Geometry check sheet. Reference: the model listing, model coordinates, mm. Coordinates: 2 decimals unless noted, no trailing zeros. Order: outer loops, then holes, each group sorted by start corner. A loop starts at its lowest first (then second) coordinate and runs counter-clockwise, first axis right, second up. Notation, with made-up numbers: (85.5, 7.5) - (129.5, 7.5) arc R31 cw to (129.5, 40.5) - close; hole circle Ø8 at (-37.75, 20). An arc over 180 degrees is marked (long way). Use CSV: the item, a comma, the result in double quotes. Start each with the question number.
1) Sectioned sample at A-A, the plane z = 7. Count the separate pieces of the cut face and the enclosed holes in it, and give its area (3 significant figures).
2) Depth check by flat-ended pin: P1, Ø1.9, axis at y = 668, z = 7.5, coming from the -X side; P2, Ø3.5, axis at x = -10.32, y = 357.19, coming from the -Z side; P3, Ø3, axis at x = 34.5, z = 3, coming from the +Y side; P4, Ø2, axis at x = -44, z = 10.5, coming from the +Y side. Enter the tip coordinate at first touch or a pass-through.
3) Sectioned sample at B-B, the plane y = 82.5. Record the cut outline in (x, z) (3 decimals), and give its area (3 significant figures).
4) Thickness scan on probe 1 along Y at (x, z) = (-18, 10); probe 2 along X at (y, z) = (237, 3) (3 decimals); probe 3 along X at (y, z) = (62, 6.25). Record the ranges inside material, lowest first. Write a range as [from, to].
from build123d import *

# Parameters (mm, degrees)
F1_DEPTH = 12.7
F2_SIZE  = 3.175
F3_R     = 2.15265
F4_DEPTH = 12.7


with BuildPart() as f1:
    # F0 (on Top) → F1 (new body)
    with BuildSketch(Plane.XY):
        with BuildLine():
            Line((-38.1, 38.1), (-38.1, 0))
            ThreePointArc((-38.1, 0), (0, -38.1), (38.1, 0))
            Line((38.1, 0), (38.1, 38.1))
            ThreePointArc((38.1, 38.1), (39.550095, 45.390119), (43.679616, 51.570384))
            Line((43.679616, 51.570384), (92.30064, 100.191409))
            ThreePointArc((92.30064, 100.191409), (99.183175, 110.49185), (101.6, 122.642049))
            Line((101.6, 122.642049), (101.6, 563.157951))
            ThreePointArc((101.6, 563.157951), (99.183175, 575.30815), (92.30064, 585.608591))
            Line((92.30064, 585.608591), (43.679616, 634.229616))
            ThreePointArc((43.679616, 634.229616), (39.550095, 640.409881), (38.1, 647.7))
            Line((38.1, 647.7), (38.1, 685.8))
            ThreePointArc((38.1, 685.8), (0, 723.9), (-38.1, 685.8))
            Line((-38.1, 685.8), (-38.1, 647.7))
            ThreePointArc((-38.1, 647.7), (-39.550095, 640.409881), (-43.679616, 634.229616))
            Line((-43.679616, 634.229616), (-92.30064, 585.608591))
            ThreePointArc((-92.30064, 585.608591), (-99.183175, 575.30815), (-101.6, 563.157951))
            Line((-101.6, 563.157951), (-101.6, 122.642049))
            ThreePointArc((-101.6, 122.642049), (-99.183175, 110.49185), (-92.30064, 100.191409))
            Line((-92.30064, 100.191409), (-43.679616, 51.570384))
            ThreePointArc((-43.679616, 51.570384), (-39.550095, 45.390119), (-38.1, 38.1))
        make_face()
    extrude(amount=F1_DEPTH)

    # F2
    f2_edges = [f1.edges().sort_by_distance(p)[0] for p in [
        (-39.550095, 45.390119, 0),
        (-38.1, 19.05, 0),
        (0, -38.1, 0),
        (38.1, 19.05, 0),
        (39.550095, 45.390119, 0),
        (67.990128, 75.880896, 0),
        (99.183175, 110.49185, 0),
        (101.6, 342.9, 0),
        (99.183175, 575.30815, 0),
        (67.990128, 609.919104, 0),
        (39.550095, 640.409881, 0),
        (38.1, 666.75, 0),
        (0, 723.9, 0),
        (-38.1, 666.75, 0),
        (-39.550095, 640.409881, 0),
        (-67.990128, 609.919104, 0),
        (-99.183175, 575.30815, 0),
        (-101.6, 342.9, 0),
        (-99.183175, 110.49185, 0),
        (-67.990128, 75.880896, 0),
        (-39.550095, 45.390119, 12.7),
        (-38.1, 19.05, 12.7),
        (0, -38.1, 12.7),
        (38.1, 19.05, 12.7),
        (39.550095, 45.390119, 12.7),
        (67.990128, 75.880896, 12.7),
        (99.183175, 110.49185, 12.7),
        (101.6, 342.9, 12.7),
        (99.183175, 575.30815, 12.7),
        (67.990128, 609.919104, 12.7),
        (39.550095, 640.409881, 12.7),
        (38.1, 666.75, 12.7),
        (0, 723.9, 12.7),
        (-38.1, 666.75, 12.7),
        (-39.550095, 640.409881, 12.7),
        (-67.990128, 609.919104, 12.7),
        (-99.183175, 575.30815, 12.7),
        (-101.6, 342.9, 12.7),
        (-99.183175, 110.49185, 12.7),
        (-67.990128, 75.880896, 12.7),
    ]]
    chamfer(f2_edges, length=F2_SIZE)

    # F3 (on face) → F4 (cut, through all)
    with BuildSketch(Plane(origin=(0, 0, 0), x_dir=(1, 0, 0), z_dir=(0, 0, -1))):
        with Locations((10.31875, -700.0875)):
            Circle(F3_R)
        with Locations((10.31875, -671.5125)):
            Circle(F3_R)
        with Locations((-10.31875, -671.5125)):
            Circle(F3_R)
        with Locations((-10.31875, -700.0875)):
            Circle(F3_R)
        with Locations((10.31875, -55.402948)):
            Circle(F3_R)
        with Locations((10.31875, -26.827948)):
            Circle(F3_R)
        with Locations((-10.31875, -55.402948)):
            Circle(F3_R)
        with Locations((-10.31875, -26.827948)):
            Circle(F3_R)
        with Locations((10.31875, -357.1875)):
            Circle(F3_R)
        with Locations((10.31875, -328.6125)):
            Circle(F3_R)
        with Locations((-10.31875, -328.6125)):
            Circle(F3_R)
        with Locations((-10.31875, -357.1875)):
            Circle(F3_R)
    extrude(amount=-F4_DEPTH, mode=Mode.SUBTRACT)


solid = f1.part
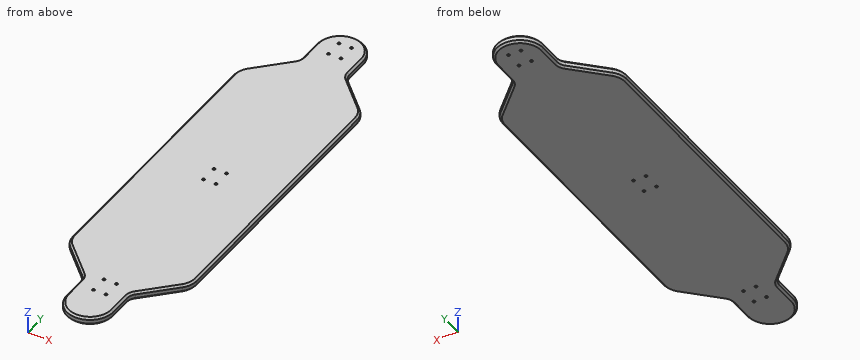
Evaluation:
1,separate pieces,"1"
1,enclosed holes,"12"
1,area,"124,000 mm²"
2,P1,"x = -38.1"
2,P2,"through"
2,P3,"y = 704.82"
2,P4,"y = 634.26"
3,outline,"(-74.609, 3.175) - (-70.119, 0) - (70.119, 0) - (74.609, 3.175) - (74.609, 9.525) - (70.119, 12.7) - (-70.119, 12.7) - (-74.609, 9.525) - close"
3,area,"1,870 mm²"
4,probe 1,"[-33.04, 718.84]"
4,probe 2,"[-101.425, 101.425]"
4,probe 3,"[-54.11, 54.11]"
